The drawing under review shows one solid part. Ordinate dimensions are in mm from its lowest x, y, z. Coordinates: 2 decimals unless noted, no trailing zeros. Loops run counter-clockwise (first coordinate to the right, second up) from the corner with the lowest first, then second, coordinate; pieces in that order, holes last. Notation, with made-up numbers: M 17.25,61 L 45.25,61 A27 cw 45.25,85 Z; hole C -2.75,46.5 d10. An arc over 180 degrees is marked long. Put each result on its own line as item: value.
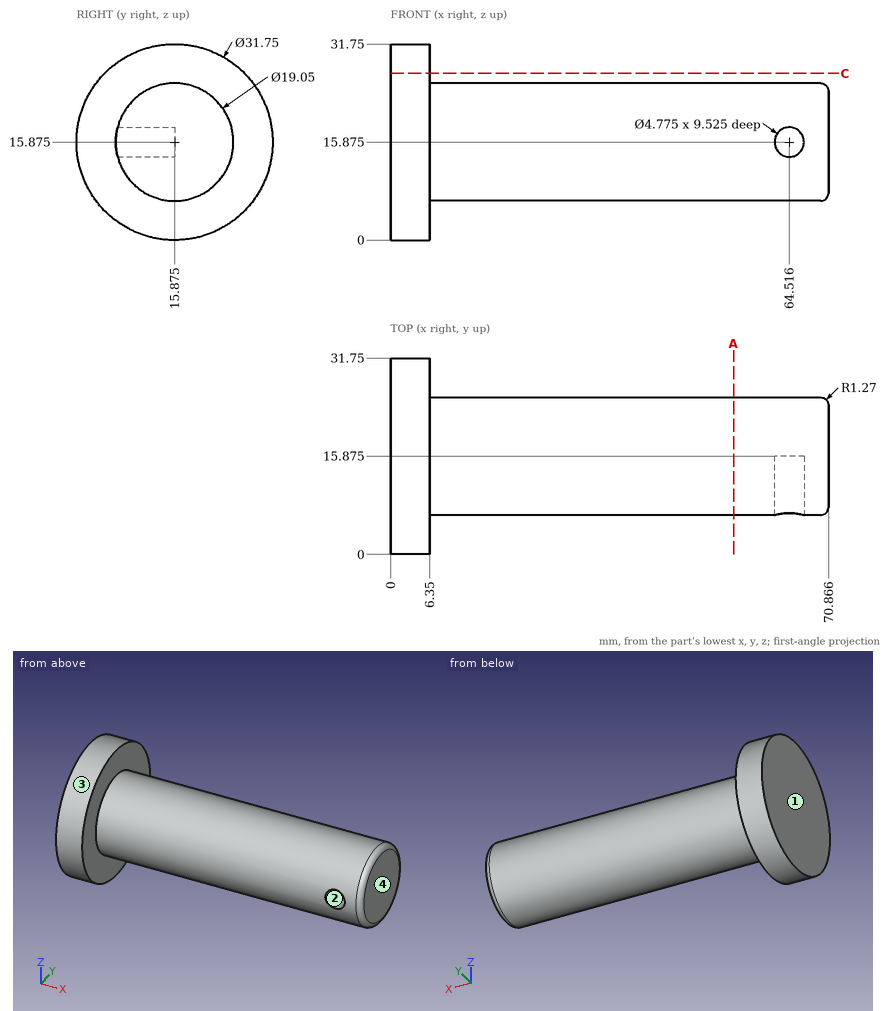
(1) Add section C-C (z = 27). Write out the cut boundary in (x, y), plus the area to 3 significant figures.
Determined:
outline: M 0,4.55 L 6.35,4.55 L 6.35,27.2 L 0,27.2 Z
area: 144 mm^2
(2) Wall thickness on line 1 along X through (y, z) = (21.5, 4.5); line 2 along X through (y, z) = (9.5, 14.5) (1 decimal); line 3 along Z through (x, y) = (65.5, 14.5): over which ranges is each line inside the solid? List them lowest first. Write a range as [from, to].
Determined:
line 1: x = [0, 6.35]
line 2: x = [0, 62.6], [66.5, 70.9]
line 3: z = [6.45, 13.7], [18.05, 25.3]
(3) For pin 1 (5.5 mm diameter, centred on x = 65, z = 16.5, fed in from -Y); pin 2 (3 mm diameter, centred on x = 56.5, z = 9, fed in from +Y); pin 3 (4 mm diameter, centred on x = 64.516, z = 15.875, fed in from -Y) (3 decimals), all flat-tipped, find the tip position at first contact; note any pin that passes through.
Determined:
pin 1: stops at y = 6.35
pin 2: stops at y = 23.74
pin 3: stops at y = 15.875
(4) Add section A-A (x = 55.5). Write out the cut boundary in (y, z) (3 decimals), plus the area to 3 significant figures.
Determined:
outline: C 15.875,15.875 d19.05
area: 285 mm^2
(5) Draft analysis for pull direction X (two halves, no side actions). For the marked faces 1, 2, 3 and 4, state which applies: +X half, -X half, draft (parallel to the pull), parting line (faces both ways), or undercut.
Determined:
face 1: -X half
face 2: undercut
face 3: draft
face 4: +X half
